Could you check a few things on this model? Use its own coordinates, in mm. Face numbers are marked on the shaded views. A direction names the side the tool comes from. Round coordinates to 2 decimals unless told otherwise and drop trailing zeros. Order: outer loops, then holes, each group sorted by start corner. A loop starts at its lowest first (then second) coordinate and runs counter-clockwise, first axis right, second up. Notation, with made-up numbers: (33.25, 66.25) - (85.25, 66.25) arc R15 ccw to (85.25, 76.25) - close; hole circle Ø11 at (44.25, -34.5). An arc over 180 degrees is marked (long way). Return JSON: item names as keys, results as strings. Group by question number.
from build123d import *

# Parameters (mm, degrees)
CYLINDER003_R     = 3
CYLINDER003_DEPTH = 10
ARRAY001_COUNT    = 8
CYLINDER002_R     = 10
CYLINDER002_DEPTH = 30
CYLINDER001_R     = 15
CYLINDER001_DEPTH = 15
CYLINDER_R        = 30
CYLINDER_DEPTH    = 5


with BuildPart() as array001:
    # Cylinder003 → Cylinder003 (new body)
    with BuildSketch(Plane(origin=(22, 0, -3), x_dir=(1, 0, 0), z_dir=(0, 0, 1))):
        Circle(CYLINDER003_R)
    extrude(amount=CYLINDER003_DEPTH)

    # Array001: Array001 ×8 about axis
    array001_axis = Axis((0, 0, 0), (0, 0, 1))


with BuildPart() as array001_1:
    add(array001.part)
    for i in range(1, ARRAY001_COUNT):
        add(array001.part.rotate(array001_axis, i * 360 / ARRAY001_COUNT))


with BuildPart() as cilindre002:
    # Cylinder002 → Cylinder002 (new body)
    with BuildSketch(Plane.XY.offset(-4)):
        Circle(CYLINDER002_R)
    extrude(amount=CYLINDER002_DEPTH)


with BuildPart() as cilindre001:
    # Cylinder001 → Cylinder001 (new body)
    with BuildSketch(Plane.XY):
        Circle(CYLINDER001_R)
    extrude(amount=CYLINDER001_DEPTH)


with BuildPart() as cut001:
    # Cylinder → Cylinder (new body)
    with BuildSketch(Plane.XY):
        Circle(CYLINDER_R)
    extrude(amount=CYLINDER_DEPTH)

    # Fusion: union Cilindre001
    add(cilindre001.part)

    # Cut: cut Cilindre002
    add(cilindre002.part, mode=Mode.SUBTRACT)

    # Cut001: cut Array001
    add(array001_1.part, mode=Mode.SUBTRACT)


solid = cut001.part
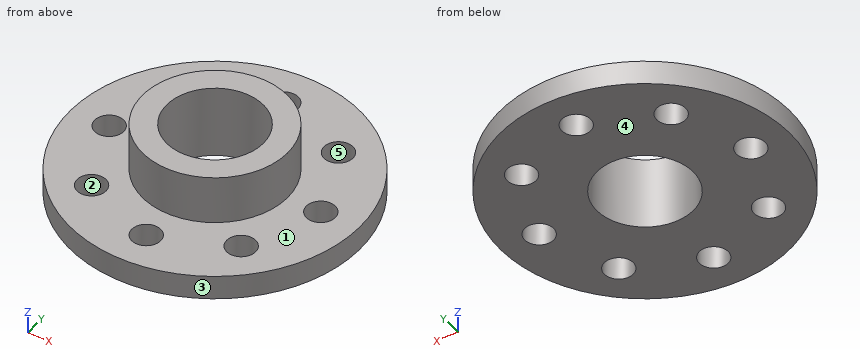
1) We'd pull the mould along Y, two halves only. Please class the marked faces 3, 4 and 5: +Y half, -Y half, draft (parallel to the pull), parting line (faces both ways), or undercut.
2) If I drill on line 1 along Y through (x, z) = (-17, 2.25); line 2 along Z through (x, y) = (-25.5, -4.5); line 3 along Y through (x, z) = (-21.5, 3.75), over which ranges is the centre line in solid material (lowest first)? Write a range as from..to.
3) I want a section at A-A, the plane y = 0. List the corners of the cut face in (x, z) for me, plus the area to 3 significant figures.
4) Will these pins go through, and if not, where does the flat tip stop? pin 1 (4 mm diameter, centred on y = 14.5, z = 2, fed in from -X); pin 2 (5 mm diameter, centred on x = 9, z = 6.5, fed in from +Y); pin 3 (3.5 mm diameter, centred on x = 15.56, y = 15.56, fed in from +Z); pin 4 (9.5 mm diameter, centred on x = -22, y = 0, fed in from +Z).
5) For the marked faces 1 and 2, which set-ups out of +Z, -Z, +X, -X, +Y, -Y let a thin tool reach every point of the face, with its end or its side?
6) I want a section at C-C, the plane y = -22. List the corners of the cut face in (x, z) for me, plus the area to 3 significant figures.
Outcome:
{
 "1": {"face 3": "parting line", "face 4": "draft", "face 5": "undercut"},
 "2": {"line 1": "-24.72..-18.19, -12.93..12.93, 18.19..24.72", "line 2": "0..5", "line 3": "-20.92..-2.96, 2.96..20.92"},
 "3": {"outline": "(-30, 0) - (-25, 0) - (-25, 5) - (-30, 5) - close; (-19, 0) - (-10, 0) - (-10, 15) - (-15, 15) - (-15, 5) - (-19, 5) - close; (10, 0) - (19, 0) - (19, 5) - (15, 5) - (15, 15) - (10, 15) - close; (25, 0) - (30, 0) - (30, 5) - (25, 5) - close", "area": "240 mm^2"},
 "4": {"pin 1": "x = -27.27", "pin 2": "y = 29.17", "pin 3": "through", "pin 4": "z = 5"},
 "5": {"face 1": "+Z", "face 2": "+Z, -Z"},
 "6": {"outline": "(-20.4, 0) - (-3, 0) - (-3, 5) - (-20.4, 5) - close; (3, 0) - (20.4, 0) - (20.4, 5) - (3, 5) - close", "area": "174 mm^2"}
}
